Geometry check sheet. Reference: the model listing, model coordinates, mm. Give positions to 0.01 mm unless a question says otherwise; leave off trailing zeros. Write each loop counter-clockwise with the first axis right and the second up, starting at its lowest first coordinate (ties: lowest second). Pieces come first, ordered by that corner, then holes. Notation, with made-up numbers: (51.5, -22.75) - (98.5, -22.75) arc R24 ccw to (98.5, -10.75) - close; hole circle Ø7 at (-20, 55). An arc over 180 degrees is marked (long way). Use a Markdown table: item, result.
```python
from build123d import *

# Parameters (mm, degrees)
SKETCH1_R           = 30
BOSS_EXTRUDE6_DEPTH = 81
SKETCH3_W           = 20
SKETCH3_H           = 12
CUT_EXTRUDE1_DEPTH  = 40.5
SKETCH4_W           = 15
SKETCH4_H           = 10
CUT_EXTRUDE2_DEPTH  = 40.5


with BuildPart() as part:
    # Sketch1 → Boss-Extrude6 (new body)
    with BuildSketch(Plane.XY):
        Circle(SKETCH1_R)
    extrude(amount=BOSS_EXTRUDE6_DEPTH)

    # Sketch3 → Cut-Extrude1 (cut, symmetric)
    with BuildSketch(Plane(origin=(0, 0, 0), x_dir=(1, 0, 0), z_dir=(0, 1, 0))):
        with Locations((0, -22.411705079)):
            Rectangle(SKETCH3_W, SKETCH3_H)
    extrude(amount=CUT_EXTRUDE1_DEPTH, both=True, mode=Mode.SUBTRACT)

    # Sketch4 → Cut-Extrude2 (cut, symmetric)
    with BuildSketch(Plane(origin=(0, 0, 0), x_dir=(1, 0, 0), z_dir=(0, 1, 0))):
        with Locations((0, -70.806519959)):
            Rectangle(SKETCH4_W, SKETCH4_H)
    extrude(amount=CUT_EXTRUDE2_DEPTH, both=True, mode=Mode.SUBTRACT)

    # Mirror1: part across plane


with BuildPart() as part_1:
    add(part.part)
    add(part.part.mirror(Plane.XY))


solid = part_1.part
```
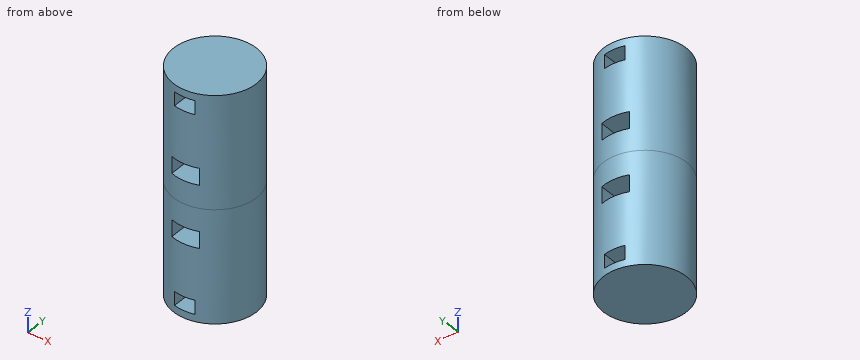
1) Section check A-A on x = 0. Record the boundary of the cut face in (y, z).
Working result:
| item | result |
|---|---|
| outline | (-30, -81) - (30, -81) - (30, -75.81) - (-30, -75.81) - close; (-30, -65.81) - (30, -65.81) - (30, -28.41) - (-30, -28.41) - close; (-30, -16.41) - (30, -16.41) - (30, 16.41) - (-30, 16.41) - close; (-30, 28.41) - (30, 28.41) - (30, 65.81) - (-30, 65.81) - close; (-30, 75.81) - (30, 75.81) - (30, 81) - (-30, 81) - close |
2) Section check D-D on z = 52. Record the boundary of the cut face in (x, y), then the cut area to 3 significant figures.
Working result:
| item | result |
|---|---|
| outline | circle Ø60 at (0, 0) |
| area | 2,830 mm² |
3) Depth check by flat-ended pin: P1, Ø5, axis at y = -7.5, z = 69, coming from the -X side; P2, Ø1, axis at y = 7, z = 4, coming from the -X side; P3, Ø6, axis at x = 0, z = -22.5, coming from the +Y side; P4, Ø4, axis at x = 1, z = 43, coming from the +Y side. Enter the tip coordinate at first touch or a pass-through.
Working result:
| item | result |
|---|---|
| P1 | stops at x = -29.58 |
| P2 | stops at x = -29.29 |
| P3 | passes through |
| P4 | stops at y = 30 |
4) Section check B-B on y = 0. Record the boundary of the cut face in (x, z).
Working result:
| item | result |
|---|---|
| outline | (-30, -81) - (30, -81) - (30, 81) - (-30, 81) - close; hole (-10, -28.41) - (10, -28.41) - (10, -16.41) - (-10, -16.41) - close; hole (-10, 16.41) - (10, 16.41) - (10, 28.41) - (-10, 28.41) - close; hole (-7.5, -75.81) - (7.5, -75.81) - (7.5, -65.81) - (-7.5, -65.81) - close; hole (-7.5, 65.81) - (7.5, 65.81) - (7.5, 75.81) - (-7.5, 75.81) - close |
5) Material ranges on L1, parallel to Z at x = 2, y = 6; L2, parallel to X at y = -25, z = -25.5; L3, parallel to X at y = -24.5, z = -70.5, recorded low to high. Write a range as from..to.
Working result:
| item | result |
|---|---|
| L1 | z = -81..-75.81, -65.81..-28.41, -16.41..16.41, 28.41..65.81, 75.81..81 |
| L2 | x = -16.58..-10, 10..16.58 |
| L3 | x = -17.31..-7.5, 7.5..17.31 |
6) Section check C-C on y = 7.5. Record the boundary of the cut face in (x, z).
Working result:
| item | result |
|---|---|
| outline | (-29.05, -81) - (29.05, -81) - (29.05, 81) - (-29.05, 81) - close; hole (-10, -28.41) - (10, -28.41) - (10, -16.41) - (-10, -16.41) - close; hole (-10, 16.41) - (10, 16.41) - (10, 28.41) - (-10, 28.41) - close; hole (-7.5, -75.81) - (7.5, -75.81) - (7.5, -65.81) - (-7.5, -65.81) - close; hole (-7.5, 65.81) - (7.5, 65.81) - (7.5, 75.81) - (-7.5, 75.81) - close |
